Read the model definition and answer for the solid it produces. Units are mm, in the model's axes. Face numbers are marked on the shaded views. Coordinates: 2 decimals unless noted, no trailing zeros. Order: outer loops, then holes, each group sorted by start corner. A loop starts at its lowest first (then second) coordinate and runs counter-clockwise, first axis right, second up. Notation, with made-up numbers: (81, 78) -> (92, 78) arc R16 cw to (92, 106) -> close; hole circle Ø8 at (39.5, 32). An arc over 180 degrees is marked (long way). Answer as a JSON object with one key per item and string values. Group by question number.
1) Section D-D on x = 25.5 is taken. Determine the outline of the cut face in (y, z).
2) Consider L1, parallel to X at y = -14.8, z = 0; L2, parallel to Y at x = 78, z = 0; L3, parallel to Z at x = 127, y = 14.65. Determine where each line is inside the solid, lowest interval first.
3) Given pin 1 (8 mm diameter, centred on x = 67.5, z = 10.5, fed in from -Y); pin 2 (3 mm diameter, centred on x = 129.5, z = 7.5, fed in from +Y); pin 3 (1.5 mm diameter, centred on x = 65, y = 6, fed in from +Z), each flat-ended and moving along its own axis, determine where each tip first touches the part or whether it passes through.
4) Section C-C on z = -1 is taken. Determine the outline of the cut face in (x, y).
5) Determine the mould class of the marked faces 1 and 2 for opening direction Y: released by +Y, released by -Y, zero draft, split by the parting line, or undercut.
6) Section B-B on x = 127 is taken. Determine the outline of the cut face in (y, z).
7) Section A-A on y = 0 is taken. Determine the outline of the cut face in (x, z).
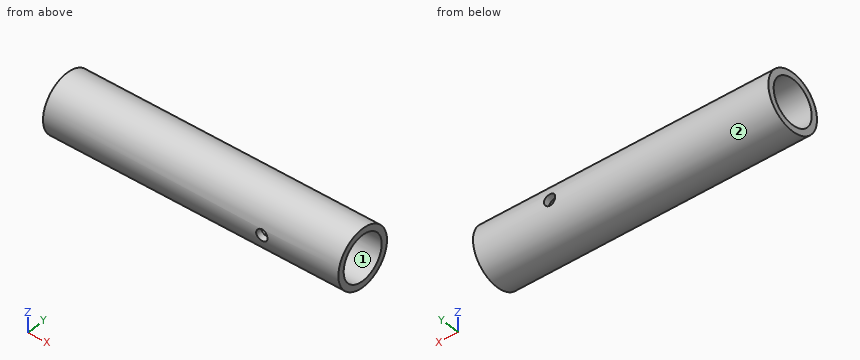
from build123d import *

# Parameters (mm, degrees)
SKETCH1_R               = 16.7005
SKETCH1_R_2             = 13.0683
BOSS_EXTRUDE1_DEPTH     = 254
CUT_EXTRUDE2_DEPTH      = 256.095694594
CUT_EXTRUDE2_DEPTH_BACK = 256.095694594
SKETCH3_R               = 3.2639
CUT_EXTRUDE4_START      = -82.55
SKETCH4_R               = 16.7005
CUT_EXTRUDE4_DEPTH      = 82.55


with BuildPart() as part:
    # Sketch1 → Boss-Extrude1 (new body)
    with BuildSketch(Plane(origin=(0, 0, 0), x_dir=(0, 0, -1), z_dir=(1, 0, 0))):
        Circle(SKETCH1_R)
        Circle(SKETCH1_R_2, mode=Mode.SUBTRACT)
    extrude(amount=BOSS_EXTRUDE1_DEPTH)

    # Sketch3 → Cut-Extrude2 (cut, two sides: drawn at the far end of the back side and taken through both)
    with BuildSketch(Plane(origin=(0, 0, 0), x_dir=(1, 0, 0), z_dir=(0, 1, 0)).offset(-CUT_EXTRUDE2_DEPTH_BACK)):
        with Locations(Location((127, 0, 0), (0, 0, 270))):
            Circle(SKETCH3_R)
    extrude(amount=CUT_EXTRUDE2_DEPTH + CUT_EXTRUDE2_DEPTH_BACK, mode=Mode.SUBTRACT)

    # Sketch4 → Cut-Extrude4 (cut)
    with BuildSketch(Plane(origin=(254, 0, 0), x_dir=(0, 0, -1), z_dir=(1, 0, 0)).offset(CUT_EXTRUDE4_START)):
        Circle(SKETCH4_R)
    extrude(amount=CUT_EXTRUDE4_DEPTH, mode=Mode.SUBTRACT)


solid = part.part
Worked answers:
{
 "1": {"outline": "circle Ø33.4 at (0, 0); hole circle Ø26.14 at (0, 0)"},
 "2": {"L1": "x = 0 to 123.74, 130.26 to 171.45", "L2": "y = -16.7 to -13.07, 13.07 to 16.7", "L3": "z = -8.02 to -3.26, 3.26 to 8.02"},
 "3": {"pin 1": "stops at y = -15.38", "pin 2": "stops at y = 15.59", "pin 3": "stops at z = 15.85"},
 "4": {"outline": "(0, -16.67) -> (123.89, -16.67) -> (123.89, -13.03) -> (0, -13.03) -> close; (0, 13.03) -> (123.89, 13.03) -> (123.89, 16.67) -> (0, 16.67) -> close; (130.11, -16.67) -> (171.45, -16.67) -> (171.45, -13.03) -> (130.11, -13.03) -> close; (130.11, 13.03) -> (171.45, 13.03) -> (171.45, 16.67) -> (130.11, 16.67) -> close"},
 "5": {"face 1": "undercut", "face 2": "split by the parting line"},
 "6": {"outline": "(-16.38, -3.26) arc R16.7 ccw to (16.38, -3.26) -> (12.65, -3.26) arc R13.07 cw to (-12.65, -3.26) -> close; (-16.38, 3.26) -> (-12.65, 3.26) arc R13.07 cw to (12.65, 3.26) -> (16.38, 3.26) arc R16.7 ccw to start"},
 "7": {"outline": "(0, -16.7) -> (171.45, -16.7) -> (171.45, -13.07) -> (0, -13.07) -> close; (0, 13.07) -> (171.45, 13.07) -> (171.45, 16.7) -> (0, 16.7) -> close"}
}
